```python
from build123d import *

# Parameters (mm, degrees)
F0_W      = 192
F0_H      = 242
F1_DEPTH  = 1
F3_D      = 110
F5_D      = 5
F6_W      = 15
F6_H      = 178
F7_DEPTH  = 1
F8_R      = 5
F9_W      = 4
F9_H      = 10
F10_DEPTH = 1
F11_R     = 1.99999


# Not quite as in the source:
# - a fillet or chamfer is up to 0.001 mm smaller than in the source, because OpenCascade refuses the exact size


with BuildPart() as f1:
    # F0 (on Front) → F1 (new body)
    with BuildSketch(Plane.XZ):
        with Locations((96, 121)):
            Rectangle(F0_W, F0_H)
    extrude(amount=F1_DEPTH)

    # F3 (through all)
    with Locations(Plane.XZ.offset(1)):
        with Locations((96, 181), (96, 61)):
            Hole(F3_D / 2)

    # F5 (through all)
    with Locations(Plane.XZ.offset(1)):
        with Locations((43.5, 233.5), (148.5, 233.5), (43.5, 128.5), (148.5, 128.5), (43.5, 113.5), (148.5, 113.5), (43.5, 8.5), (148.5, 8.5)):
            Hole(F5_D / 2)

    # F6 (on face) → F7 (cut)
    with BuildSketch(Plane.XZ.offset(1)):
        with Locations((7.5, 121)):
            Rectangle(F6_W, F6_H)
        with Locations((184.5, 121)):
            Rectangle(F6_W, F6_H)
    extrude(amount=-F7_DEPTH, mode=Mode.SUBTRACT)

    # F8
    f8_edges = [f1.edges().sort_by_distance(p)[0] for p in [
        (0, -0.5, 210),
        (0, -0.5, 242),
        (0, -0.5, 32),
        (0, -0.5, 0),
        (192, -0.5, 32),
        (192, -0.5, 0),
        (192, -0.5, 242),
        (192, -0.5, 210),
    ]]
    fillet(f8_edges, radius=F8_R)

    # F9 (on face) → F10 (cut)
    with BuildSketch(Plane.XZ.offset(1)):
        with Locations((7.5, 226)):
            Rectangle(F9_W, F9_H)
        with Locations((184.5, 226)):
            Rectangle(F9_W, F9_H)
        with Locations((7.5, 16)):
            Rectangle(F9_W, F9_H)
        with Locations((184.5, 16)):
            Rectangle(F9_W, F9_H)
    extrude(amount=-F10_DEPTH, mode=Mode.SUBTRACT)

    # F11 (radius 2 in the source; OpenCascade refuses exactly that, so slightly less here)
    f11_edges = [f1.edges().sort_by_distance(p)[0] for p in [
        (9.5, -0.5, 231),
        (5.5, -0.5, 231),
        (5.5, -0.5, 221),
        (9.5, -0.5, 221),
        (182.5, -0.5, 231),
        (186.5, -0.5, 231),
        (182.5, -0.5, 221),
        (186.5, -0.5, 221),
        (182.5, -0.5, 21),
        (186.5, -0.5, 21),
        (186.5, -0.5, 11),
        (182.5, -0.5, 11),
        (5.5, -0.5, 21),
        (9.5, -0.5, 21),
        (9.5, -0.5, 11),
        (5.5, -0.5, 11),
    ]]
    fillet(f11_edges, radius=F11_R)


solid = f1.part
```
For this review, take the finished solid that the model builds, in its own axes (mm). A direction names the side the tool comes from. Give positions to 0.01 mm unless a question says otherwise; leave off trailing zeros. Order: outer loops, then holes, each group sorted by start corner. A loop starts at its lowest first (then second) coordinate and runs counter-clockwise, first axis right, second up.
1) Take a section at A-A (z = 61). Give the boundary of the cut face in (x, y), then the cut area to 3 significant figures.
2) The part is to be moulded in two halves that separate along Z. For faces 1 (the face through (1.5, -0.49, 211.43)), 2 (the face through (95, 0, 123)), 3 (the face through (190.5, -0.51, 240.57)), 4 (the face through (1.43, -0.51, 1.5)), say which applies: released by +Z, released by -Z, zero draft, split by the parting line, or undercut.
3) Take a section at D-D (y = -0.8). State how many separate pieces and enclosed holes the cut face has, then the cut area to 3 significant figures.
4) Take a section at C-C (x = 122). Give the boundary of the cut face in (y, z), then the cut area to 3 significant figures.
5) For faces 5 (the face through (1.43, -0.49, 30.5)), 6 (the face through (41.19, -0.49, 7.54)), 7 (the face through (190.57, -0.49, 211.5)), list the 3-axis set-ups (+Z, -Z, +X, -X, +Y, -Y) from which the entire face can be reached by the end or side of a thin tool; tool diameter is ignored.
6) Take a section at B-B (x = 148.5). Give the boundary of the cut face in (y, z), then the cut area to 3 significant figures.
7) Insertion check: pin 1 (4 mm diameter, centred on x = 43.5, z = 128.5, fed in from +Y). The pin has a flat end and moves straight along its axis. Give the tip position at first contact, or say it passes through.
8) Wall thickness on line 1 (Z direction, x = 119, y = -0.75); line 2 (Z direction, x = 96, y = -0.8); line 3 (X direction, y = -0.5, z = 45): over which ranges is each line inside the solid? List them lowest first.
Derived:
1. outline: (15, -1) - (41, -1) - (41, 0) - (15, 0) - close; (151, -1) - (177, -1) - (177, 0) - (151, 0) - close
1. area: 52.0 mm2
2. face 1: undercut
2. face 2: zero draft
2. face 3: released by +Z
2. face 4: released by -Z
3. separate pieces: 1
3. enclosed holes: 14
3. area: 21,800 mm2
4. outline: (-1, 0) - (0, 0) - (0, 12.53) - (-1, 12.53) - close; (-1, 109.47) - (0, 109.47) - (0, 132.53) - (-1, 132.53) - close; (-1, 229.47) - (0, 229.47) - (0, 242) - (-1, 242) - close
4. area: 48.1 mm2
5. face 5: -X, +Y, -Y
5. face 6: +Y, -Y
5. face 7: +X, +Y, -Y
6. outline: (-1, 0) - (0, 0) - (0, 6) - (-1, 6) - close; (-1, 11) - (0, 11) - (0, 44.61) - (-1, 44.61) - close; (-1, 77.39) - (0, 77.39) - (0, 111) - (-1, 111) - close; (-1, 116) - (0, 116) - (0, 126) - (-1, 126) - close; (-1, 131) - (0, 131) - (0, 164.61) - (-1, 164.61) - close; (-1, 197.39) - (0, 197.39) - (0, 231) - (-1, 231) - close; (-1, 236) - (0, 236) - (0, 242) - (-1, 242) - close
6. area: 156 mm2
7. pin 1: passes through
8. line 1: z = 0 to 11.04, 110.96 to 131.04, 230.96 to 242
8. line 2: z = 0 to 6, 116 to 126, 236 to 242
8. line 3: x = 15 to 43.38, 148.62 to 177
